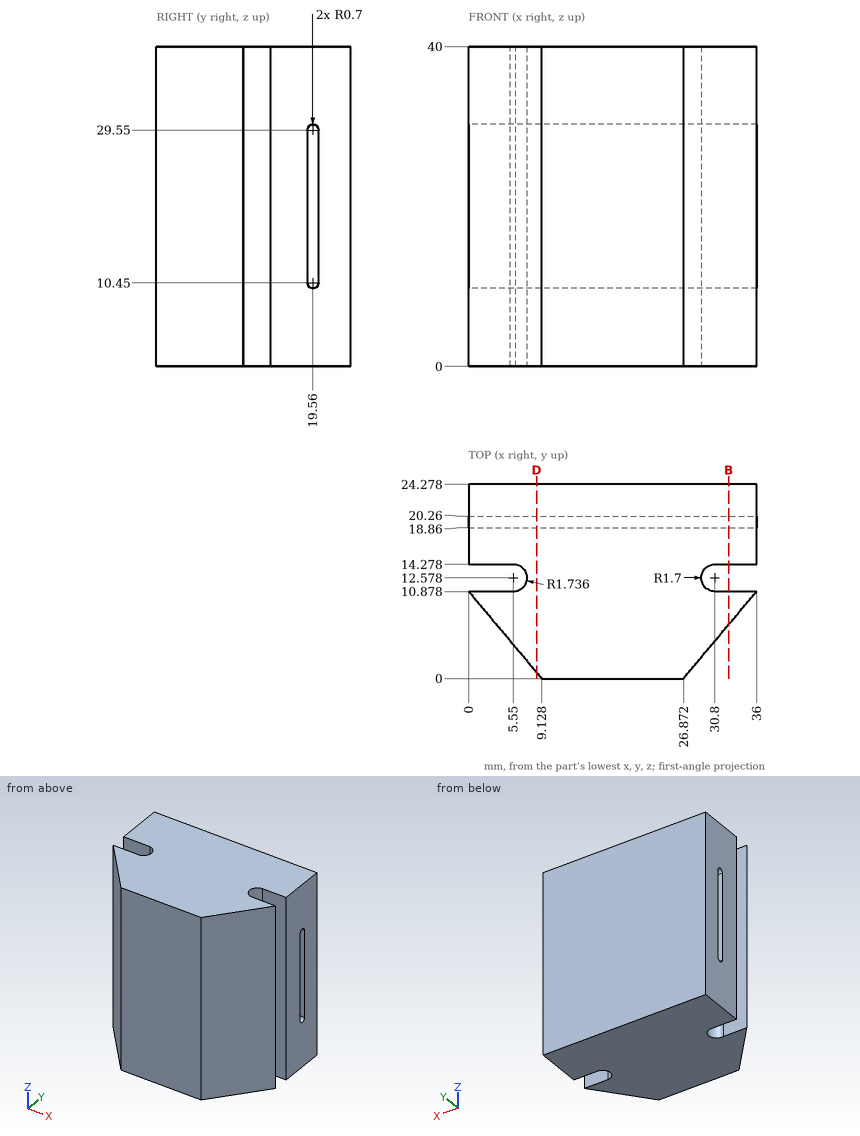
Verification items for this drawing (mm, ordinates from the low corner). Coordinates: 2 decimals unless noted, no trailing zeros. Write each loop counter-clockwise with the first axis right and the second up, starting at its lowest first coordinate (ties: lowest second). Pieces come first, ordered by that corner, then holes. Notation, with made-up numbers: M 58.5,-34 L 75.5,-34 A29 ccw 75.5,1 Z; hole C -6.5,-2.75 d9. An arc over 180 degrees is marked long. One line per item, written item: value. Start each with the question number.
(1) Depth check by flat-ended pin: pin 1 (1 mm diameter, centred on y = 19, z = 22.5, fed in from -X); pin 2 (1.6 mm diameter, centred on x = 34.5, z = 20, fed in from -Y) (1 decimal); pin 3 (4 mm diameter, centred on y = 7.5, z = 28, fed in from +X) (1 decimal); pin 4 (1.8 mm diameter, centred on x = 3.5, z = 19, fed in from -Y) (1 decimal). Enter the tip coordinate at first touch or a pass-through.
(2) Sectioned sample at B-B, the plane x = 32.5. Enter the section's corners in (y, z).
(3) Sectioned sample at D-D, the plane x = 8.5. Enter the section's corners in (y, z).
(4) Scan lines: line 1 along Y through (x, z) = (16, 26); line 2 along Y through (x, z) = (33, 19) (1 decimal); line 3 along Y through (x, z) = (7.5, 11). Record each from-to range of solid material in increasing order. Write a range as [from, to].
Filled sheet:
1. pin 1: x = 0
1. pin 2: y = 8.1
1. pin 3: x = 34.8
1. pin 4: y = 5.6
2. outline: M 6.71,0 L 10.88,0 L 10.88,40 L 6.71,40 Z; M 14.28,0 L 24.28,0 L 24.28,40 L 14.28,40 Z; hole M 18.86,10.45 A0.7 ccw 20.26,10.45 L 20.26,29.55 A0.7 ccw 18.86,29.55 Z
3. outline: M 0.75,0 L 24.28,0 L 24.28,40 L 0.75,40 Z; hole M 18.86,10.45 A0.7 ccw 20.26,10.45 L 20.26,29.55 A0.7 ccw 18.86,29.55 Z
4. line 1: [0, 18.86], [20.26, 24.28]
4. line 2: [7.3, 10.9], [14.3, 18.9], [20.3, 24.3]
4. line 3: [1.94, 18.86], [20.26, 24.28]
